Could you check a few things on this model? Use its own coordinates, in mm. Give positions to 0.01 mm unless a question says otherwise; leave off trailing zeros. Loops run counter-clockwise (first coordinate to the right, second up) from the corner with the lowest first, then second, coordinate; pieces in that order, holes last. Notation, with made-up numbers: (-5.5, 50.5) -> (40.5, 50.5) arc R35 ccw to (40.5, 86.5) -> close; hole circle Ø9 at (-22.5, 6.5). An arc over 180 degrees is marked (long way). Write item = value, one per line. Start each with the question number.
1) I need wall thicknesses on probe 1 along Y at (x, z) = (0, 1.8); probe 2 along X at (y, z) = (-2, 2.9); probe 3 along X at (y, z) = (-23, 1.65). Which ranges of each line are inside material? Lowest first, please. Write a range as from..to.
2) I want a section at A-A (x = 0). List the corners of the cut face in (y, z) for me.
3) If we mould it in two halves opening along X, with no side actions, what happens to faces 1 (the face through (-159.041, 0, 2)), 2 (the face through (-43, 0, 4)), 3 (the face through (-59.096, 22.605, 1.972))? For each: +X half, -X half, draft (parallel to the pull), parting line (faces both ways), or undercut.
4) I want a section at C-C (z = 2.35). Count the separate pieces of the cut face and the enclosed holes in it, and give its area (3 significant figures).
5) I want a section at B-B (y = 0). List the corners of the cut face in (x, z) for me, and give its area (3 significant figures).
from build123d import *

# Parameters (mm, degrees)
SKETCH1_W           = 235
SKETCH1_H           = 60
SKETCH1_R           = 7.1
SKETCH1_R_2         = 1.55
SKETCH1_R_3         = 2.55
BOSS_EXTRUDE1_DEPTH = 4


with BuildPart() as part:
    # Sketch1 → Boss-Extrude1 (new body)
    with BuildSketch(Plane.XY):
        with Locations((-41.541275094, 0)):
            Rectangle(SKETCH1_W, SKETCH1_H)
        with Locations((-133, 0)):
            Circle(SKETCH1_R, mode=Mode.SUBTRACT)
        with Locations((50, 0)):
            Circle(SKETCH1_R, mode=Mode.SUBTRACT)
        Circle(SKETCH1_R, mode=Mode.SUBTRACT)
        with Locations((68.451377883, -22.492652976)):
            Circle(SKETCH1_R_2, mode=Mode.SUBTRACT)
        with Locations((68.451377883, 22.492652976)):
            Circle(SKETCH1_R_2, mode=Mode.SUBTRACT)
        with Locations((-56.548622117, -22.492652976)):
            Circle(SKETCH1_R_3, mode=Mode.SUBTRACT)
        with Locations((-56.548622117, 22.492652976)):
            Circle(SKETCH1_R_3, mode=Mode.SUBTRACT)
        with Locations((-76.548622117, -22.492652976)):
            Circle(SKETCH1_R_3, mode=Mode.SUBTRACT)
        with Locations((-76.548622117, 22.492652976)):
            Circle(SKETCH1_R_3, mode=Mode.SUBTRACT)
    extrude(amount=BOSS_EXTRUDE1_DEPTH)


solid = part.part
Answer list:
q1.probe_1 = -30..-7.1, 7.1..30
q1.probe_2 = -159.04..-139.81, -126.19..-6.81, 6.81..43.19, 56.81..75.96
q1.probe_3 = -159.04..-79.05, -74.05..-59.05, -54.05..66.99, 69.92..75.96
q2.outline = (-30, 0) -> (-7.1, 0) -> (-7.1, 4) -> (-30, 4) -> close; (7.1, 0) -> (30, 0) -> (30, 4) -> (7.1, 4) -> close
q3.face_1 = -X half
q3.face_2 = draft
q3.face_3 = undercut
q4.separate_pieces = 1
q4.enclosed_holes = 9
q4.area = 13,500 mm^2
q5.outline = (-159.04, 0) -> (-140.1, 0) -> (-140.1, 4) -> (-159.04, 4) -> close; (-125.9, 0) -> (-7.1, 0) -> (-7.1, 4) -> (-125.9, 4) -> close; (7.1, 0) -> (42.9, 0) -> (42.9, 4) -> (7.1, 4) -> close; (57.1, 0) -> (75.96, 0) -> (75.96, 4) -> (57.1, 4) -> close
q5.area = 770 mm^2
